from build123d import *

# Parameters (mm, degrees)
SKETCH1_W           = 8.5
SKETCH1_H           = 5
BOSS_EXTRUDE1_DEPTH = 1.5
BOSS_EXTRUDE2_DEPTH = 2.5
SKETCH3_W           = 8.5
SKETCH3_H           = 5
BOSS_EXTRUDE3_DEPTH = 1.5
SKETCH4_R           = 1.25
CUT_EXTRUDE1_DEPTH  = 11.5


with BuildPart() as part:
    # Sketch1 → Boss-Extrude1 (new body)
    with BuildSketch(Plane(origin=(0, 0, 0), x_dir=(1, 0, 0), z_dir=(0, 1, 0))):
        Rectangle(SKETCH1_W, SKETCH1_H)
    extrude(amount=BOSS_EXTRUDE1_DEPTH)

    # Sketch2 → Boss-Extrude2 (add)
    with BuildSketch(Plane(origin=(0, 1.5, 0), x_dir=(1, 0, 0), z_dir=(0, 1, 0))):
        with BuildLine():
            Line((-0.75, -2.5), (0.75, -2.5))
            Line((0.75, -2.5), (0.75, -1.600781056))
            ThreePointArc((0.75, -1.600781056), (0, 1.76776695), (-0.75, -1.600781056))
            Line((-0.75, -1.600781056), (-0.75, -2.5))
        make_face()
    extrude(amount=BOSS_EXTRUDE2_DEPTH)

    # Sketch3 → Boss-Extrude3 (add)
    with BuildSketch(Plane(origin=(0, 4, 0), x_dir=(1, 0, 0), z_dir=(0, 1, 0))):
        Rectangle(SKETCH3_W, SKETCH3_H)
    extrude(amount=BOSS_EXTRUDE3_DEPTH)

    # Sketch4 → Cut-Extrude1 (cut)
    with BuildSketch(Plane(origin=(0, 5.5, 0), x_dir=(1, 0, 0), z_dir=(0, 1, 0))):
        Circle(SKETCH4_R)
    extrude(amount=-CUT_EXTRUDE1_DEPTH, mode=Mode.SUBTRACT)


solid = part.part
Read the model definition and answer for the solid it produces. Units are mm, in the model's axes. A direction names the side the tool comes from. Round coordinates to 2 decimals unless told otherwise and drop trailing zeros. Write each loop counter-clockwise with the first axis right and the second up, starting at its lowest first coordinate (ties: lowest second). Pieces come first, ordered by that corner, then holes.
Q1. A tool of negligible diameter and unlimited length cuts with its end or side. For faces 4 (the face through (0.75, 3, 2)), 5 (the face through (0.067, 2.732, -1.767)), 6 (the face through (-0.75, 3, 2)), from which of +Z, -Z, +X, -X, +Y, -Y can it reach the whole face along a straight path? Write none if from no direction.
Values:
face 4: +Z, +X
face 5: none
face 6: +Z, -X
Q2. Find section B-B on z = 0. Determine the outline of the cut face in (x, y).
Values:
outline: (-4.25, 0) - (-1.25, 0) - (-1.25, 5.5) - (-4.25, 5.5) - (-4.25, 4) - (-1.77, 4) - (-1.77, 1.5) - (-4.25, 1.5) - close; (1.25, 0) - (4.25, 0) - (4.25, 1.5) - (1.77, 1.5) - (1.77, 4) - (4.25, 4) - (4.25, 5.5) - (1.25, 5.5) - close
Q3. Find section C-C on y = 2.65. Determine the outline of the cut face in (x, z), and give its area (3 significant figures).
Values:
outline: (-0.75, 1.6) arc R1.77 ccw (long way) to (0.75, 1.6) - (0.75, 2.5) - (-0.75, 2.5) - close; hole circle Ø2.5 at (0, 0)
area: 6.09 mm2
Q4. Straight lines are drawn through the part: line 1 (X direction, y = 4.35, z = 0); line 2 (X direction, y = 2.7, z = 0); line 3 (Y direction, x = -2.5, z = -0.75). For each, find the intervals that lie inside material, in ascending order.
Values:
line 1: x = -4.25 to -1.25, 1.25 to 4.25
line 2: x = -1.77 to -1.25, 1.25 to 1.77
line 3: y = 0 to 1.5, 4 to 5.5
Q5. The mould has two halves that part along X. Classify faces 1 (the face through (0, 1, -2.5)), 2 (the face through (4.25, 5, 0)), 3 (the face through (-0.27, 2.79, 1.22)): released by +X, released by -X, zero draft, split by the parting line, or undercut.
Values:
face 1: zero draft
face 2: released by +X
face 3: undercut
Q6. Find section D-D on x = 0. Determine the outline of the cut face in (y, z), and give its area (3 significant figures).
Values:
outline: (0, -2.5) - (1.5, -2.5) - (1.5, -1.77) - (4, -1.77) - (4, -2.5) - (5.5, -2.5) - (5.5, -1.25) - (0, -1.25) - close; (0, 1.25) - (5.5, 1.25) - (5.5, 2.5) - (0, 2.5) - close
area: 11.9 mm2
Q7. Find section A-A on x = 2. Determine the outline of the cut face in (y, z), and give its area (3 significant figures).
Values:
outline: (0, -2.5) - (1.5, -2.5) - (1.5, 2.5) - (0, 2.5) - close; (4, -2.5) - (5.5, -2.5) - (5.5, 2.5) - (4, 2.5) - close
area: 15.0 mm2
Q8. Flat-ended cylindrical pins translate along their axes: P1, Ø1, axis at y = 2.5, z = 2, coming from the -X side; P2, Ø2, axis at x = 0, z = 0, coming from the +Y side. Find the tip coordinate at first contact, or state that the pin passes through.
Values:
P1: stops at x = -0.94
P2: passes through
